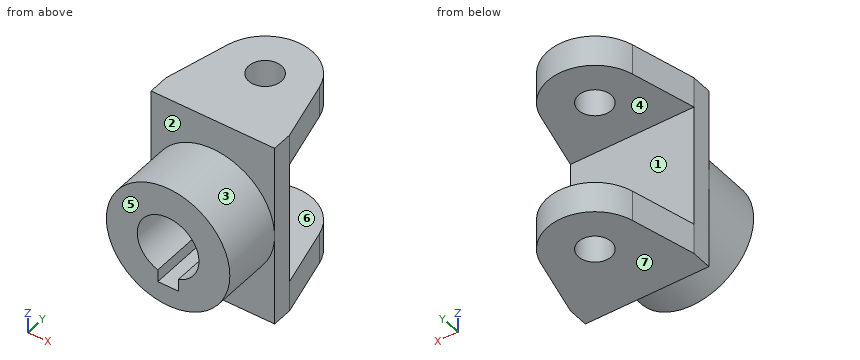
```python
from build123d import *

# Parameters (mm, degrees)
SKETCH1_R           = 15
BOSS_EXTRUDE1_DEPTH = 10
BOSS_EXTRUDE2_DEPTH = 30
SKETCH3_R           = 8
BOSS_EXTRUDE3_DEPTH = 15


with BuildPart() as part:
    # Sketch1 → Boss-Extrude1 (new body)
    # profile 1 of 5: a face of its own
    with BuildSketch(Plane(origin=(0, 0, 0), x_dir=(1, 0, 0), z_dir=(0, 1, 0))):
        with BuildLine():
            ThreePointArc((-30, -1.1e-08), (5e-09, -30), (30, 0))
            ThreePointArc((30, 0), (-5e-09, 30), (-30, -1.1e-08))
        make_face()
        with BuildLine():
            Line((5, 20.142135624), (5, 14.142135624))
            ThreePointArc((5, 14.142135624), (12.247448714, 8.660254038), (15, 0))
            ThreePointArc((15, 0), (-8.660254038, -12.247448714), (-5, 14.142135624))
            Line((-5, 14.142135624), (-5, 20.142135624))
            Line((-5, 20.142135624), (5, 20.142135624))
        make_face(mode=Mode.SUBTRACT)
    # profile 2 of 5: a face of its own
    with BuildSketch(Plane(origin=(0, 0, 0), x_dir=(1, 0, 0), z_dir=(0, 1, 0))):
        Circle(SKETCH1_R)
    # profile 3 of 5: a face of its own
    with BuildSketch(Plane(origin=(0, 0, 0), x_dir=(1, 0, 0), z_dir=(0, 1, 0))):
        with BuildLine():
            ThreePointArc((-5, 14.142135624), (0, 15), (5, 14.142135624))
            Line((5, 14.142135624), (5, 20.142135624))
            Line((5, 20.142135624), (-5, 20.142135624))
            Line((-5, 20.142135624), (-5, 14.142135624))
        make_face()
    # profile 4 of 5: a face of its own
    with BuildSketch(Plane(origin=(0, 0, 0), x_dir=(1, 0, 0), z_dir=(0, 1, 0))):
        with BuildLine():
            Line((-30, -45), (30, -45))
            Line((30, -45), (30, 0))
            ThreePointArc((30, 0), (5e-09, -30), (-30, -1.1e-08))
            Line((-30, -1.1e-08), (-30, -45))
        make_face()
    # profile 5 of 5: a face of its own
    with BuildSketch(Plane(origin=(0, 0, 0), x_dir=(1, 0, 0), z_dir=(0, 1, 0))):
        with BuildLine():
            ThreePointArc((-30, -1.1e-08), (-5e-09, 30), (30, 0))
            Line((30, 0), (30, 45))
            Line((30, 45), (-30, 45))
            Line((-30, 45), (-30, -1.1e-08))
        make_face()
    extrude(amount=BOSS_EXTRUDE1_DEPTH)

    # Sketch1_3 → Boss-Extrude2 (add)
    with BuildSketch(Plane(origin=(0, 0, 0), x_dir=(1, 0, 0), z_dir=(0, 1, 0))):
        with BuildLine():
            ThreePointArc((-30, -1.1e-08), (5e-09, -30), (30, 0))
            ThreePointArc((30, 0), (-5e-09, 30), (-30, -1.1e-08))
        make_face()
        with BuildLine():
            Line((5, 20.142135624), (5, 14.142135624))
            ThreePointArc((5, 14.142135624), (12.247448714, 8.660254038), (15, 0))
            ThreePointArc((15, 0), (-8.660254038, -12.247448714), (-5, 14.142135624))
            Line((-5, 14.142135624), (-5, 20.142135624))
            Line((-5, 20.142135624), (5, 20.142135624))
        make_face(mode=Mode.SUBTRACT)
    extrude(amount=-BOSS_EXTRUDE2_DEPTH)

    # Sketch3 → Boss-Extrude3 (add)
    with BuildSketch(Plane.XY.offset(45)):
        with BuildLine():
            Line((30, 10), (22.306028796, 40.607234555))
            ThreePointArc((22.306028796, 40.607234555), (0, 58), (-22.306028796, 40.607234555))
            Line((-22.306028796, 40.607234555), (-30, 10))
            Line((-30, 10), (30, 10))
        make_face()
        with Locations((0, 35)):
            Circle(SKETCH3_R, mode=Mode.SUBTRACT)
    boss_extrude3 = extrude(amount=-BOSS_EXTRUDE3_DEPTH)

    # Mirror1: Boss-Extrude3 across plane
    add(boss_extrude3.mirror(Plane.XY))


solid = part.part
```
Could you check a few things on this model? Use its own coordinates, in mm. Face numbers are marked on the shaded views. A direction names the side the tool comes from. Round coordinates to 2 decimals unless told otherwise and drop trailing zeros. Write each loop counter-clockwise with the first axis right and the second up, starting at its lowest first coordinate (ties: lowest second). Pieces come first, ordered by that corner, then holes.
(1) Suppose I cut it at C-C on z = -33. Write out the boundary of the cut face in (x, y).
Findings below:
outline: (-30, 0) - (30, 0) - (30, 10) - (22.31, 40.61) arc R23 ccw to (-22.31, 40.61) - (-30, 10) - close; hole circle Ø16 at (0, 35)
(2) Suppose I cut it at B-B on y = 35. Write out the boundary of the cut face in (x, z).
Findings below:
outline: (-23.72, -45) - (-8, -45) - (-8, -30) - (-23.72, -30) - close; (-23.72, 30) - (-8, 30) - (-8, 45) - (-23.72, 45) - close; (8, -45) - (23.72, -45) - (23.72, -30) - (8, -30) - close; (8, 30) - (23.72, 30) - (23.72, 45) - (8, 45) - close
(3) For pin 1 (12 mm diameter, centred on y = 38.5, z = 28, fed in from -X); pin 2 (2 mm diameter, centred on x = -23.5, z = -19.5, fed in from +Y); pin 3 (5 mm diameter, centred on x = 0.5, y = -18.5, fed in from +Z), each with a flat end and sliding along its axis, tell me the tip position at first contact or that it passes through.
Findings below:
pin 1: stops at x = -24.26
pin 2: stops at y = 10
pin 3: stops at z = 30
(4) If I drill on probe 1 along Y at (x, z) = (0, -34); probe 2 along Z at (x, y) = (-8, 51.5); probe 3 along Y at (x, z) = (-7, -24), over which ranges is the centre line in solid material (lowest first)?
Findings below:
probe 1: y = 0 to 27, 43 to 58
probe 2: z = -45 to -30, 30 to 45
probe 3: y = -30 to 10
(5) Thinking about a two-plate mould opening in Z: for the marked faces 4, 5, 6 and 7, which applies, +Z half, -Z half, draft (parallel to the pull), parting line (faces both ways), or undercut?
Findings below:
face 4: undercut
face 5: draft
face 6: undercut
face 7: -Z half
(6) Suppose I cut it at D-D on y = 48. Write out the boundary of the cut face in (x, z).
Findings below:
outline: (-18.97, -45) - (18.97, -45) - (18.97, -30) - (-18.97, -30) - close; (-18.97, 30) - (18.97, 30) - (18.97, 45) - (-18.97, 45) - close
(7) Which directions (+Z, -Z, +X, -X, +Y, -Y) give clear straight access to the entire face, cutting with the end or side of a thin tool? Please do the marked faces 1, 2 and 3.
Findings below:
face 1: +X, -X, +Y
face 2: +Z, -Y
face 3: -Y
(8) Suppose I cut it at A-A on x = 0. Write out the boundary of the cut face in (y, z).
Findings below:
outline: (-30, -30) - (0, -30) - (0, -45) - (27, -45) - (27, -30) - (10, -30) - (10, 30) - (27, 30) - (27, 45) - (0, 45) - (0, 30) - (-30, 30) - (-30, 15) - (0, 15) - (0, -20.14) - (-30, -20.14) - close; (43, -45) - (58, -45) - (58, -30) - (43, -30) - close; (43, 30) - (58, 30) - (58, 45) - (43, 45) - close
